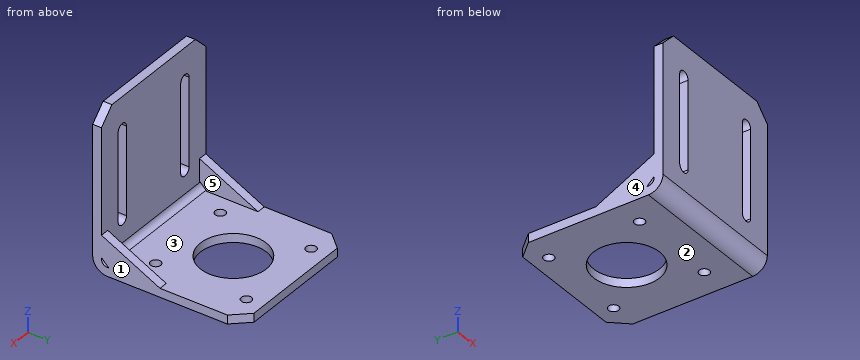
from build123d import *

# Parameters (mm, degrees)
ESQUISSE1_R        = 11.25
ESQUISSE1_R_2      = 1.75
BOSS_EXTRU_1_DEPTH = 3
BOSS_EXTRU_2_DEPTH = 3
CONG_1_R           = 2
CONG_2_R           = 5
BOSS_EXTRU_3_DEPTH = 3
BOSS_EXTRU_4_START = -50
BOSS_EXTRU_4_DEPTH = 3


with BuildPart() as part:
    # Esquisse1 → Boss.-Extru.1 (new body)
    with BuildSketch(Plane.XY):
        Polygon((-20, 51.5), (20, 51.5), (25, 46), (25, 0), (-25, 0), (-25, 46), align=None)
        with Locations((0, 30.25)):
            Circle(ESQUISSE1_R, mode=Mode.SUBTRACT)
        with Locations((15.5, 45.75)):
            Circle(ESQUISSE1_R_2, mode=Mode.SUBTRACT)
        with Locations((15.5, 14.75)):
            Circle(ESQUISSE1_R_2, mode=Mode.SUBTRACT)
        with Locations((-15.5, 14.75)):
            Circle(ESQUISSE1_R_2, mode=Mode.SUBTRACT)
        with Locations((-15.5, 45.75)):
            Circle(ESQUISSE1_R_2, mode=Mode.SUBTRACT)
    extrude(amount=BOSS_EXTRU_1_DEPTH)

    # Esquisse2 → Boss.-Extru.2 (add)
    with BuildSketch(Plane.XZ):
        Polygon((-20, 54), (20, 54), (25, 49), (25, 0), (-25, 0), (-25, 49), align=None)
        with BuildLine():
            Line((17, 43), (17, 13))
            ThreePointArc((17, 13), (15, 11), (13, 13))
            Line((13, 13), (13, 43))
            ThreePointArc((13, 43), (15, 45), (17, 43))
        make_face(mode=Mode.SUBTRACT)
        with BuildLine():
            Line((-17, 43), (-17, 13))
            ThreePointArc((-17, 13), (-15, 11), (-13, 13))
            Line((-13, 13), (-13, 43))
            ThreePointArc((-13, 43), (-15, 45), (-17, 43))
        make_face(mode=Mode.SUBTRACT)
    extrude(amount=-BOSS_EXTRU_2_DEPTH)

    # Congé1
    cong_1_edges = [part.edges().sort_by_distance(p)[0] for p in [
        (0, 3, 3),
    ]]
    fillet(cong_1_edges, radius=CONG_1_R)

    # Congé2
    cong_2_edges = [part.edges().sort_by_distance(p)[0] for p in [
        (0, 0, 0),
    ]]
    fillet(cong_2_edges, radius=CONG_2_R)

    # Esquisse3 → Boss.-Extru.3 (add)
    with BuildSketch(Plane.ZY.offset(25)):
        Polygon((13, 3), (3, 23), (3, 5.5), (5.5, 3), align=None)
    extrude(amount=-BOSS_EXTRU_3_DEPTH)

    # Esquisse3<3> → Boss.-Extru.4 (add)
    with BuildSketch(Plane.ZY.offset(25).offset(BOSS_EXTRU_4_START)):
        Polygon((13, 3), (3, 23), (3, 5.5), (5.5, 3), align=None)
    extrude(amount=BOSS_EXTRU_4_DEPTH)


solid = part.part
Check sheet for the modelled part. Datum: model origin and axes. Units: mm. Face numbers are marked on the shaded views. A direction names the side the tool comes from. Coordinates: 2 decimals unless noted, no trailing zeros. Write each loop counter-clockwise with the first axis right and the second up, starting at its lowest first coordinate (ties: lowest second). Pieces come first, ordered by that corner, then holes. Notation, with made-up numbers: M 44.5,-12 L 92.5,-12 A27 cw 92.5,15 Z; hole C -32,-23 d3. An arc over 180 degrees is marked long. Answer as CSV lines item,"result".
Q1. Mould release check, pull along X, two halves, no side actions. Record for the marked faces 1, 2 and 3: released by +X, released by -X, zero draft, split by the parting line, or undercut.
Check result:
face 1,"released by +X"
face 2,"zero draft"
face 3,"undercut"
Q2. Cross-section at B-B (y = 37). Record the boundary of the cut face in (x, z), then the cut area to 3 significant figures.
Check result:
outline,"M -25,0 L -9,0 L -9,3 L -25,3 Z; M 9,0 L 25,0 L 25,3 L 9,3 Z"
area,"96.0 mm^2"
Q3. Cross-section at D-D (z = 7). Record the boundary of the cut face in (x, y).
Check result:
outline,"M -25,0 L 25,0 L 25,15 L 22,15 L 22,3 L -22,3 L -22,15 L -25,15 Z"
Q4. Cross-section at C-C (x = 3.5). Record the boundary of the cut face in (y, z).
Check result:
outline,"M 0,5 A5 ccw 5,0 L 19.56,0 L 19.56,3 L 5,3 A2 cw 3,5 L 3,54 L 0,54 Z; M 40.94,0 L 51.5,0 L 51.5,3 L 40.94,3 Z"
Q5. Go/stop test with flat-tipped pins: pin 1 (1.5 mm diameter, centred on x = 17, y = 5.5, fed in from +Z); pin 2 (14.5 mm diameter, centred on x = 2.5, z = 34, fed in from +Y). Record where each tip stops, or that it passes through.
Check result:
pin 1,"z = 3.02"
pin 2,"y = 3"
Q6. Set-up check for the marked faces 4 and 5: record each of +Z, -Z, +X, -X, +Y, -Y from which the full face is reachable in a straight line by a thin tool's end or side.
Check result:
face 4,"+Z, -Z, -X, +Y, -Y"
face 5,"+Z, +Y"
Q7. Cross-section at A-A (z = 23.5). Record the boundary of the cut face in (x, y).
Check result:
outline,"M -25,0 L -17,0 L -17,3 L -25,3 Z; M -13,0 L 13,0 L 13,3 L -13,3 Z; M 17,0 L 25,0 L 25,3 L 17,3 Z"
Q8. Material ranges on probe 1 along Y at (x, z) = (-15, 1); probe 2 along Y at (x, z) = (-15.5, 0.8); probe 3 along Z at (x, y) = (-10.5, 14), recorded low to high. Write a range as from..to.
Check result:
probe 1,"2..13.07, 16.43..44.07, 47.43..51.5"
probe 2,"2.29..13, 16.5..44, 47.5..51.5"
probe 3,"0..3"
